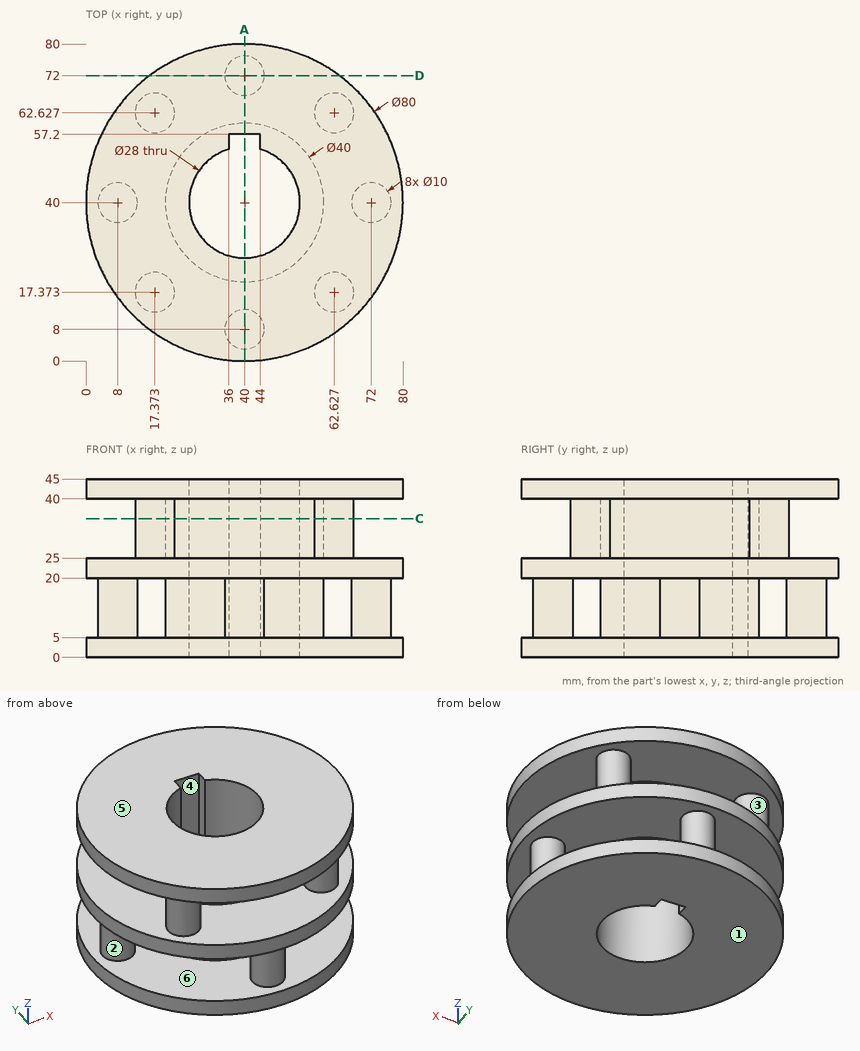
For this review, use the dimensioned drawing (mm, ordinates from the lowest corner) and the shaded views. A direction names the side the tool comes from. Give positions to 0.01 mm unless a question says otherwise; leave off trailing zeros. Order: outer loops, then holes, each group sorted by start corner. A loop starts at its lowest first (then second) coordinate and runs counter-clockwise, first axis right, second up. Notation, with made-up numbers: M -21,-24 L 33,-24 A19 cw 33,-14 Z; hole C -39,-39.5 d11. An arc over 180 degrees is marked long. Use one line per item in the form item = value. Start each with the question number.
Item 1: For the marked faces 4, 5 and 6, list the 3-axis set-ups (+Z, -Z, +X, -X, +Y, -Y) from which the entire face can be reached by the end or side of a thin tool; tool diameter is ignored.
Item 2: We need section D-D on y = 72. Give the boundary of the cut face in (x, z), plus the area to 3 significant figures.
Item 3: The part is to be moulded in two halves that separate along Y. For the marked faces 1, 2 and 3, say which applies: pulls with the +Y half, pulls with the -Y half, needs draft (parallel to the pull), parting line crosses it, or undercut.
Item 4: To check wall thickness, follow line 1 along Z through (x, y) = (35, 12.5); line 2 along Y through (x, z) = (35.5, 17.5) (1 decimal); line 3 along Y through (x, z) = (40, 29). State the ranges of each line that lie inside material, in increasing order. Write a range as from..to.
Item 5: Insertion check: pin 1 Ø4 at (x, z) = (70, 32) entering from +Y; pin 2 Ø6.5 at (x, z) = (40, 18) entering from -Y; pin 3 Ø3 at (y, z) = (55.5, 21.5) entering from +X; pin 4 Ø1.1 at (y, z) = (55, 24) entering from -X. Each pin has a flat end and moves straight along its axis. Give the tip position at first contact, or say it passes through.
Item 6: We need section A-A on x = 40. Give the number of separate pieces and of enclosed holes in the cut face, plus the area to 3 significant figures.
Item 7: We need section C-C on z = 35. Give the boundary of the cut face in (x, y).
Completed:
q1.face_4 = +Z, -Z
q1.face_5 = +Z, +X, -X, +Y, -Y
q1.face_6 = none
q2.outline = M 16,0 L 64,0 L 64,5 L 45,5 L 45,20 L 64,20 L 64,25 L 16,25 L 16,20 L 35,20 L 35,5 L 16,5 Z; M 16,40 L 64,40 L 64,45 L 16,45 Z
q2.area = 870 mm²
q3.face_1 = needs draft
q3.face_2 = parting line crosses it
q3.face_3 = undercut
q4.line_1 = 0..5, 20..25, 40..45
q4.line_2 = 5.8..10.2, 20.5..26.7, 53.3..59.5, 69.8..74.2
q4.line_3 = 20..26, 57.2..60
q5.pin_1 = through
q5.pin_2 = 0
q5.pin_3 = 77.47
q5.pin_4 = 2.7
q6.separate_pieces = 2
q6.enclosed_holes = 2
q6.area = 1,300 mm²
q7.outline = C 17.37,17.37 d10; C 17.37,62.63 d10; C 40,40 d40; C 62.63,17.37 d10; C 62.63,62.63 d10; hole M 36,53.42 A14 ccw long 44,53.42 L 44,57.2 L 36,57.2 Z
